from build123d import *

# Parameters (mm, degrees)
ESQUISSE1_W             = 16
ESQUISSE1_H             = 5
BOSS_EXTRU_1_DEPTH      = 65
BOSS_EXTRU_3_DEPTH      = 65
ESQUISSE2_R             = 2.5
ENL_V_MAT_EXTRU_1_DEPTH = 66.76473219
CONG_1_R                = 4
CONG_2_R                = 1


with BuildPart() as part:
    # Esquisse1 → Boss.-Extru.1 (new body)
    with BuildSketch(Plane.XY):
        Rectangle(ESQUISSE1_W, ESQUISSE1_H)
    extrude(amount=BOSS_EXTRU_1_DEPTH)

    # Esquisse4 → Boss.-Extru.3 (add)
    with BuildSketch(Plane.XY.offset(65)):
        Polygon((-1.75, -3.5), (1.75, -3.5), (2.75, -2.5), (-2.75, -2.5), align=None)
    extrude(amount=-BOSS_EXTRU_3_DEPTH)

    # Esquisse2 → Enlèv. mat.-Extru.1 (cut, through all)
    with BuildSketch(Plane(origin=(0, 2.5, 0), x_dir=(1, 0, 0), z_dir=(0, 1, 0))):
        with Locations(Location((0, -7.5, 0), (0, 0, 270))):
            Circle(ESQUISSE2_R)
        with Locations(Location((0, -57.5, 0), (0, 0, 225.572995999))):
            Circle(ESQUISSE2_R)
    extrude(amount=-ENL_V_MAT_EXTRU_1_DEPTH, mode=Mode.SUBTRACT)

    # Congé1
    cong_1_edges = [part.edges().sort_by_distance(p)[0] for p in [
        (8, 0, 65),
        (8, 0, 0),
    ]]
    fillet(cong_1_edges, radius=CONG_1_R)

    # Congé2
    cong_2_edges = [part.edges().sort_by_distance(p)[0] for p in [
        (-8, 0, 65),
        (-8, 0, 0),
    ]]
    fillet(cong_2_edges, radius=CONG_2_R)


solid = part.part
Verification items for the finished model (mm, model axes). A direction names the side the tool comes from. Give positions to 0.01 mm unless a question says otherwise; leave off trailing zeros. Loops run counter-clockwise (first coordinate to the right, second up) from the corner with the lowest first, then second, coordinate; pieces in that order, holes last. Notation, with made-up numbers: (86, -40) - (128, -40) arc R19 cw to (128, -9) - close; hole circle Ø4 at (31, 19). An arc over 180 degrees is marked (long way). Write each question's results on one line, items separated by ' | '.
1) Tool access check on faces 4 (the flat face through (-5, -2.5, 32)), 5 (the flat face through (8, 0, 32)), 6 (the flat face through (5, -2.5, 32)). Record the directions out of +Z, -Z, +X, -X, +Y, -Y that give a thin tool (end or side, any length) a straight path to the whole face; none if there is none.
Solution:
face 4: +Z, -Z, -X, -Y | face 5: +Z, -Z, +X, +Y, -Y | face 6: +Z, -Z, +X, -Y
2) Depth check by flat-ended pin: P1, Ø3, axis at x = 0, z = 57.5, coming from the +Y side; P2, Ø4, axis at x = 4, z = 17.5, coming from the -Y side; P3, Ø3, axis at x = -5, z = 10.5, coming from the -Y side; P4, Ø4, axis at x = -4.5, z = 20, coming from the -Y side. Enter the tip coordinate at first touch or a pass-through.
Solution:
P1: through | P2: y = -3.25 | P3: y = -2.5 | P4: y = -2.75
3) Sectioned sample at A-A on x = 0. Record the boundary of the cut face in (y, z), plus the area to 3 significant figures.
Solution:
outline: (-3.5, 0) - (2.5, 0) - (2.5, 5) - (-3.5, 5) - close; (-3.5, 10) - (2.5, 10) - (2.5, 55) - (-3.5, 55) - close; (-3.5, 60) - (2.5, 60) - (2.5, 65) - (-3.5, 65) - close | area: 330 mm2
4) Mould release check, pull along X, two halves, no side actions. Record for faces 1 (the cylindrical face through (6.797, 0.035, 1.141)), 2 (the cylindrical face through (2.48, -0.46, 7.17)), 3 (the flat face through (-2, 0, 65)): pulls with the +X half, pulls with the -X half, needs draft (parallel to the pull), parting line crosses it, or undercut.
Solution:
face 1: pulls with the +X half | face 2: undercut | face 3: needs draft
5) Sectioned sample at D-D on z = 43.5. Record the boundary of the cut face in (x, y), plus the area to 3 significant figures.
Solution:
outline: (-8, -2.5) - (-2.75, -2.5) - (-1.75, -3.5) - (1.75, -3.5) - (2.75, -2.5) - (8, -2.5) - (8, 2.5) - (-8, 2.5) - close | area: 84.5 mm2
6) Sectioned sample at C-C on y = 0.05. Record the boundary of the cut face in (x, z), plus the area to 3 significant figures.
Solution:
outline: (-8, 1) arc R1 ccw to (-7, 0) - (4, 0) arc R4 ccw to (8, 4) - (8, 61) arc R4 ccw to (4, 65) - (-7, 65) arc R1 ccw to (-8, 64) - close; hole circle Ø5 at (0, 7.5); hole circle Ø5 at (0, 57.5) | area: 993 mm2
7) Material ranges on L1, parallel to Z at x = 0, y = -1.6; L2, parallel to X at y = -1.35, z = 57.5; L3, parallel to Z at x = 2, y = -2.3, recorded low to high. Write a range as from..to.
Solution:
L1: 0..5, 10..55, 60..65 | L2: -8..-2.5, 2.5..8 | L3: 0..6, 9..56, 59..65
8) Sectioned sample at B-B on z = 57.5. Record the boundary of the cut face in (x, y).
Solution:
outline: (-8, -2.5) - (-2.75, -2.5) - (-2.5, -2.75) - (-2.5, 2.5) - (-8, 2.5) - close; (2.5, -2.75) - (2.75, -2.5) - (8, -2.5) - (8, 2.5) - (2.5, 2.5) - close
